Here's how the part is built. I have some questions about the finished solid (model axes, mm). Face numbers are marked on the shaded views. A direction names the side the tool comes from. Give positions to 0.01 mm unless a question says otherwise; leave off trailing zeros. Write each loop counter-clockwise with the first axis right and the second up, starting at its lowest first coordinate (ties: lowest second). Pieces come first, ordered by that corner, then holes. Notation, with made-up numbers: (26, 54.5) - (85, 54.5) arc R20 cw to (85, 64.5) - close; hole circle Ø6 at (38, 1.5). An arc over 180 degrees is marked (long way). Use a Markdown table: item, result.
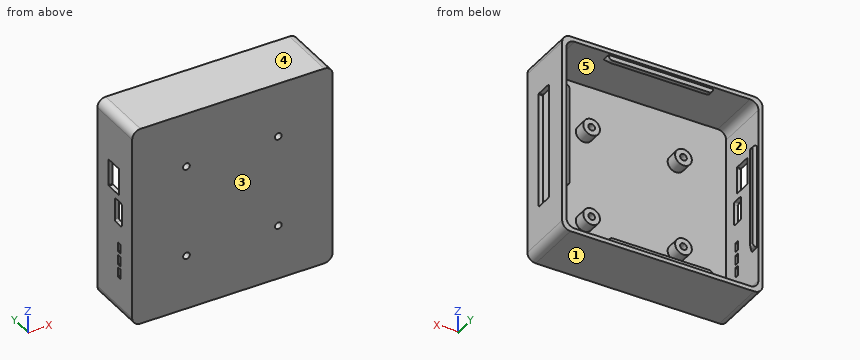
```python
from build123d import *

# Parameters (mm, degrees)
SKETCH_1_W               = 96
SKETCH_1_H               = 96
EXTRUDE_1_DEPTH          = 28
SKETCH_3_W               = 92
SKETCH_3_H               = 92
CUT_EXTRUDE_1_DEPTH      = 26
FILLET_1_R               = 4
FILLET_2_R               = 4
SKETCH_4_R               = 4
EXTRUDE_2_DEPTH          = 6
SKETCH_5_R               = 1.6
CUT_EXTRUDE_2_DEPTH      = 8
SKETCH_6_W               = 12.999999928
SKETCH_6_H               = 8.49999995
SKETCH_6_W_2             = 4.700000191
SKETCH_6_H_2             = 1.900000077
SKETCH_6_W_3             = 4.600000187
SKETCH_6_H_3             = 1.849687021
SKETCH_6_W_4             = 4.500000183
SKETCH_6_W_5             = 11.544018717
SKETCH_6_H_4             = 5.642342208
CUT_EXTRUDE_3_DEPTH      = 2
FILLET_3_R               = 0.4
SKETCH_7_W               = 55.768080965
SKETCH_7_H               = 8.199999866
CUT_EXTRUDE_4_DEPTH      = 2
FILLET_4_R               = 0.5
FILLET_5_R               = 1
SKETCH_8_W               = 50
SKETCH_8_H               = 2
EXTRUDE_3_DEPTH          = 2.2
FILLET_6_R               = 2
PATTERN_CIRCULAR_1_COUNT = 4
FILLET_7_R               = 2
CHAMFER_START            = 23
CHAMFER_1_DEPTH          = 50
CHAMFER_START_2          = 22.8
CHAMFER_1_2_DEPTH        = 2
CHAMFER_2_DEPTH          = 50
CHAMFER_2_2_DEPTH        = 2
CHAMFER_3_DEPTH          = 50
CHAMFER_3_2_DEPTH        = 2
CHAMFER_4_DEPTH          = 50
CHAMFER_4_2_DEPTH        = 2


with BuildPart() as part:
    # 草图1 → 凸台-拉伸1 (new body)
    with BuildSketch(Plane(origin=(0, 0, 0), x_dir=(1, 0, 0), z_dir=(0, 1, 0))):
        with Locations((48, -48)):
            Rectangle(SKETCH_1_W, SKETCH_1_H)
    extrude(amount=EXTRUDE_1_DEPTH)

    # 草图3 → 切除-拉伸1 (cut)
    with BuildSketch(Plane(origin=(0, 28, 0), x_dir=(1, 0, 0), z_dir=(0, 1, 0))):
        with Locations((48, -48)):
            Rectangle(SKETCH_3_W, SKETCH_3_H)
    extrude(amount=-CUT_EXTRUDE_1_DEPTH, mode=Mode.SUBTRACT)

    # 圆角1
    fillet_1_edges = [part.edges().sort_by_distance(p)[0] for p in [
        (2, 15, 94),
        (2, 15, 2),
        (94, 15, 2),
        (94, 15, 94),
    ]]
    fillet(fillet_1_edges, radius=FILLET_1_R)

    # 圆角2
    fillet_2_edges = [part.edges().sort_by_distance(p)[0] for p in [
        (0, 14, 0),
        (96, 14, 0),
        (96, 14, 96),
        (0, 14, 96),
    ]]
    fillet(fillet_2_edges, radius=FILLET_2_R)

    # 草图4 → 凸台-拉伸2 (add)
    with BuildSketch(Plane(origin=(0, 2, 0), x_dir=(1, 0, 0), z_dir=(0, 1, 0))):
        with Locations(Location((26, -26, 0), (0, 0, 270))):
            Circle(SKETCH_4_R)
        with Locations(Location((70, -26, 0), (0, 0, 90))):
            Circle(SKETCH_4_R)
        with Locations(Location((70, -70, 0), (0, 0, 270))):
            Circle(SKETCH_4_R)
        with Locations(Location((26, -70, 0), (0, 0, 90))):
            Circle(SKETCH_4_R)
    extrude(amount=EXTRUDE_2_DEPTH)

    # 草图5 → 切除-拉伸2 (cut)
    with BuildSketch(Plane(origin=(0, 8, 0), x_dir=(1, 0, 0), z_dir=(0, 1, 0))):
        with Locations(Location((26, -26, 0), (0, 0, 270))):
            Circle(SKETCH_5_R)
        with Locations(Location((70, -26, 0), (0, 0, 270))):
            Circle(SKETCH_5_R)
        with Locations(Location((26, -70, 0), (0, 0, 270))):
            Circle(SKETCH_5_R)
        with Locations(Location((70, -70, 0), (0, 0, 270))):
            Circle(SKETCH_5_R)
    extrude(amount=-CUT_EXTRUDE_2_DEPTH, mode=Mode.SUBTRACT)

    # 草图6 → 切除-拉伸3 (cut)
    with BuildSketch(Plane.ZY):
        with Locations((65.087122174, 14.836156947)):
            Rectangle(SKETCH_6_W, SKETCH_6_H)
        with Locations((20.344696565, 10.485844036)):
            Rectangle(SKETCH_6_W_2, SKETCH_6_H_2)
        with Locations((26.390708755, 10.511000564)):
            Rectangle(SKETCH_6_W_3, SKETCH_6_H_3)
        with Locations((32.663721202, 10.485844036)):
            Rectangle(SKETCH_6_W_4, SKETCH_6_H_2)
        with Locations((49.799296419, 11.158551524)):
            Rectangle(SKETCH_6_W_5, SKETCH_6_H_4)
    extrude(amount=-CUT_EXTRUDE_3_DEPTH, mode=Mode.SUBTRACT)

    # 圆角3
    fillet_3_edges = [part.edges().sort_by_distance(p)[0] for p in [
        (1, 10.586156972, 58.58712221),
        (1, 19.086156922, 58.58712221),
        (1, 19.086156922, 71.587122138),
        (1, 10.586156972, 71.587122138),
    ]]
    fillet(fillet_3_edges, radius=FILLET_3_R)

    # 草图7 → 切除-拉伸4 (cut)
    with BuildSketch(Plane(origin=(96, 0, 0), x_dir=(0, 0, -1), z_dir=(1, 0, 0))):
        with Locations((-49.248086711, 13.186156826)):
            Rectangle(SKETCH_7_W, SKETCH_7_H)
    extrude(amount=-CUT_EXTRUDE_4_DEPTH, mode=Mode.SUBTRACT)

    # 圆角4
    fillet_4_edges = [part.edges().sort_by_distance(p)[0] for p in [
        (95, 9.086156893, 77.132127193),
        (95, 17.286156759, 77.132127193),
        (95, 17.286156759, 21.364046228),
        (95, 9.086156893, 21.364046228),
    ]]
    fillet(fillet_4_edges, radius=FILLET_4_R)

    # 圆角5
    fillet_5_edges = [part.edges().sort_by_distance(p)[0] for p in [
        (1, 8.33738042, 44.02728706),
        (1, 13.979722628, 44.02728706),
        (1, 13.979722628, 55.571305777),
        (1, 8.33738042, 55.571305777),
    ]]
    fillet(fillet_5_edges, radius=FILLET_5_R)

    # 草图8 → 凸台-拉伸3 (add)
    with BuildSketch(Plane(origin=(0, 0, 94), x_dir=(-1, 0, 0), z_dir=(0, 0, -1))):
        with Locations((-48, 25.8)):
            Rectangle(SKETCH_8_W, SKETCH_8_H)
    extrude_3 = extrude(amount=EXTRUDE_3_DEPTH)

    # 圆角6
    fillet_6_edges = [part.edges().sort_by_distance(p)[0] for p in [
        (73, 25.8, 91.8),
        (23, 25.8, 91.8),
    ]]
    fillet(fillet_6_edges, radius=FILLET_6_R)

    # 阵列(圆周)1: 凸台-拉伸3 ×4 about axis
    pattern_circular_1_axis = Axis((48, 0, 48), (0, 1, 0))
    for i in range(1, PATTERN_CIRCULAR_1_COUNT):
        add(extrude_3.rotate(pattern_circular_1_axis, i * 360 / PATTERN_CIRCULAR_1_COUNT))

    # 圆角7
    fillet_7_edges = [part.edges().sort_by_distance(p)[0] for p in [
        (91.8, 25.8, 23),
        (91.8, 25.8, 73),
        (23, 25.8, 4.2),
        (73, 25.8, 4.2),
        (4.2, 25.8, 73),
        (4.2, 25.8, 23),
    ]]
    fillet(fillet_7_edges, radius=FILLET_7_R)

    # 倒角1: read off the stored shape, not the designer's step
    # 倒角1 outline → 倒角1 (add)
    with BuildSketch(Plane.YZ.offset(CHAMFER_START)):
        Polygon((24.8, 2), (24.8, 4), (22.8, 2), align=None)
    extrude(amount=CHAMFER_1_DEPTH)

    # Chamfer 1 2 outline → Chamfer 1 2 (cut)
    with BuildSketch(Plane(origin=(0, 0, 0), x_dir=(1, 0, 0), z_dir=(0, 1, 0)).offset(CHAMFER_START_2)):
        with BuildLine():
            Line((73, -4.20000003), (73, -2.2))
            ThreePointArc((73, -2.2), (72.414213562, -3.614213562), (71, -4.2))
            Line((71, -4.2), (73, -4.20000003))
        make_face()
        with BuildLine():
            Line((23, -4.20000003), (25, -4.2))
            ThreePointArc((25, -4.2), (23.585786438, -3.614213562), (23, -2.2))
            Line((23, -2.2), (23, -4.20000003))
        make_face()
    extrude(amount=CHAMFER_1_2_DEPTH, mode=Mode.SUBTRACT)

    # 倒角2: read off the stored shape, not the designer's step
    # 倒角2 outline → 倒角2 (add)
    with BuildSketch(Plane.YZ.offset(CHAMFER_START)):
        Polygon((24.8, 94), (22.8, 94), (24.8, 92), align=None)
    extrude(amount=CHAMFER_2_DEPTH)

    # Chamfer 2 2 outline → Chamfer 2 2 (cut)
    with BuildSketch(Plane(origin=(0, 0, 0), x_dir=(1, 0, 0), z_dir=(0, 1, 0)).offset(CHAMFER_START_2)):
        with BuildLine():
            Line((23, -91.79999997), (23, -93.8))
            ThreePointArc((23, -93.8), (23.585786438, -92.385786438), (25, -91.8))
            Line((25, -91.8), (23, -91.79999997))
        make_face()
        with BuildLine():
            Line((73, -91.79999997), (71, -91.8))
            ThreePointArc((71, -91.8), (72.414213562, -92.385786438), (73, -93.8))
            Line((73, -93.8), (73, -91.79999997))
        make_face()
    extrude(amount=CHAMFER_2_2_DEPTH, mode=Mode.SUBTRACT)

    # 倒角3: read off the stored shape, not the designer's step
    # 倒角3 outline → 倒角3 (add)
    with BuildSketch(Plane.XY.offset(CHAMFER_START)):
        Polygon((94, 24.8), (92, 24.8), (94, 22.8), align=None)
    extrude(amount=CHAMFER_3_DEPTH)

    # Chamfer 3 2 outline → Chamfer 3 2 (cut)
    with BuildSketch(Plane(origin=(0, 0, 0), x_dir=(1, 0, 0), z_dir=(0, 1, 0)).offset(CHAMFER_START_2)):
        with BuildLine():
            Line((91.79999997, -73), (93.8, -73))
            ThreePointArc((93.8, -73), (92.385786438, -72.414213562), (91.8, -71))
            Line((91.8, -71), (91.79999997, -73))
        make_face()
        with BuildLine():
            Line((91.79999997, -23), (91.8, -25))
            ThreePointArc((91.8, -25), (92.385786438, -23.585786438), (93.8, -23))
            Line((93.8, -23), (91.79999997, -23))
        make_face()
    extrude(amount=CHAMFER_3_2_DEPTH, mode=Mode.SUBTRACT)

    # 倒角4: read off the stored shape, not the designer's step
    # 倒角4 outline → 倒角4 (add)
    with BuildSketch(Plane.XY.offset(CHAMFER_START)):
        Polygon((2, 24.8), (2, 22.8), (4, 24.8), align=None)
    extrude(amount=CHAMFER_4_DEPTH)

    # Chamfer 4 2 outline → Chamfer 4 2 (cut)
    with BuildSketch(Plane(origin=(0, 0, 0), x_dir=(1, 0, 0), z_dir=(0, 1, 0)).offset(CHAMFER_START_2)):
        with BuildLine():
            Line((4.20000003, -23), (2.2, -23))
            ThreePointArc((2.2, -23), (3.614213562, -23.585786438), (4.2, -25))
            Line((4.2, -25), (4.20000003, -23))
        make_face()
        with BuildLine():
            Line((4.200000031, -73), (4.2, -71))
            ThreePointArc((4.2, -71), (3.614213562, -72.414213562), (2.2, -73))
            Line((2.2, -73), (4.200000031, -73))
        make_face()
    extrude(amount=CHAMFER_4_2_DEPTH, mode=Mode.SUBTRACT)


solid = part.part
```
Item 1: I need wall thicknesses on line 1 along X through (y, z) = (5.5, 70); line 2 along X through (y, z) = (18.5, 76.5). Which ranges of each line are inside material? Lowest first, please. Write a range as [from, to].
Values:
| item | result |
|---|---|
| line 1 | x = [0, 2], [22, 24.4], [27.6, 30], [66, 68.4], [71.6, 74], [94, 96] |
| line 2 | x = [0, 2], [94, 96] |
Item 2: Will these pins go through, and if not, where does the flat tip stop? pin 1 Ø2 at (x, y) = (0.5, 10) entering from -Z; pin 2 Ø8 at (x, z) = (42.5, 30) entering from +Y; pin 3 Ø0.6 at (x, y) = (1, 10) entering from -Z.
Values:
| item | result |
|---|---|
| pin 1 | stops at z = 0.88 |
| pin 2 | stops at y = 2 |
| pin 3 | stops at z = 1.05 |
Item 3: If we section it at C-C, the plane z = 38: Write out the boundary of the cut face in (x, y).
Values:
| item | result |
|---|---|
| outline | (0, 0) - (96, 0) - (96, 9.09) - (94, 9.09) - (94, 2) - (2, 2) - (2, 22.8) - (4, 24.8) - (4.2, 24.8) - (4.2, 26.8) - (2, 26.8) - (2, 28) - (0, 28) - close; (91.8, 24.8) - (92, 24.8) - (94, 22.8) - (94, 17.29) - (96, 17.29) - (96, 28) - (94, 28) - (94, 26.8) - (91.8, 26.8) - close |
Item 4: Thinking about a two-plate mould opening in Y: for the marked faces 1, 2 and 3, which applies, +Y half, -Y half, draft (parallel to the pull), parting line (faces both ways), or undercut?
Values:
| item | result |
|---|---|
| face 1 | draft |
| face 2 | undercut |
| face 3 | -Y half |
Item 5: If we section it at A-A, the plane y = 5.75: Count the separate pieces of the cut face and the enclosed holes in it, plus the area to 3 significant figures.
Values:
| item | result |
|---|---|
| separate pieces | 5 |
| enclosed holes | 5 |
| area | 921 mm2 |
Item 6: If we section it at B-B, the plane y = 21: Write out the boundary of the cut face in (x, z), plus the area to 3 significant figures.
Values:
| item | result |
|---|---|
| outline | (0, 4) arc R4 ccw to (4, 0) - (92, 0) arc R4 ccw to (96, 4) - (96, 92) arc R4 ccw to (92, 96) - (4, 96) arc R4 ccw to (0, 92) - close; hole (2, 6) arc R4 ccw to (6, 2) - (90, 2) arc R4 ccw to (94, 6) - (94, 90) arc R4 ccw to (90, 94) - (6, 94) arc R4 ccw to (2, 90) - close |
| area | 752 mm2 |
Item 7: For the marked faces 4 and 5, which set-ups out of +Z, -Z, +X, -X, +Y, -Y let a thin tool reach every point of the face, with its end or its side?
Values:
| item | result |
|---|---|
| face 4 | +Z, +X, -X, +Y, -Y |
| face 5 | none |
